from build123d import *

# Parameters (mm, degrees)
PAD_DEPTH       = 6
POCKET_DEPTH    = 5
SKETCH002_R     = 2.25
SKETCH002_R_2   = 1.6
PAD001_DEPTH    = 4
POCKET001_DEPTH = 10


with BuildPart() as part:
    # Sketch → Pad (new body)
    with BuildSketch(Plane.XY):
        with BuildLine():
            Line((3, 0), (62, 0))
            ThreePointArc((62, 0), (64.12132, 0.87868), (65, 3))
            Line((65, 3), (65, 27))
            ThreePointArc((65, 27), (64.12132, 29.12132), (62, 30))
            Line((62, 30), (3, 30))
            ThreePointArc((3, 30), (0.87868, 29.12132), (0, 27))
            Line((0, 27), (0, 3))
            ThreePointArc((0, 3), (0.87868, 0.87868), (3, 0))
        make_face()
    extrude(amount=PAD_DEPTH)

    # Sketch001 → Pocket (cut)
    with BuildSketch(Plane.XY):
        with BuildLine():
            Line((1, 27), (1, 3))
            ThreePointArc((1, 3), (1.585786, 1.585786), (3, 1))
            Line((3, 1), (62, 1))
            ThreePointArc((62, 1), (63.414214, 1.585786), (64, 3))
            Line((64, 3), (64, 27))
            ThreePointArc((64, 27), (63.414214, 28.414214), (62, 29))
            Line((62, 29), (3, 29))
            ThreePointArc((3, 29), (1.585786, 28.414214), (1, 27))
        make_face()
    extrude(amount=POCKET_DEPTH, mode=Mode.SUBTRACT)

    # Sketch002 → Pad001 (join)
    with BuildSketch(Plane.XY.offset(1)):
        with Locations((62.25, 27.3)):
            Circle(SKETCH002_R)
        with Locations((62.25, 27.3)):
            Circle(SKETCH002_R_2, mode=Mode.SUBTRACT)
        with Locations((2.75, 27.3)):
            Circle(SKETCH002_R)
        with Locations((2.75, 27.3)):
            Circle(SKETCH002_R_2, mode=Mode.SUBTRACT)
        with Locations((2.75, 2.7)):
            Circle(SKETCH002_R)
        with Locations((2.75, 2.7)):
            Circle(SKETCH002_R_2, mode=Mode.SUBTRACT)
        with Locations((62.25, 2.7)):
            Circle(SKETCH002_R)
        with Locations((62.25, 2.7)):
            Circle(SKETCH002_R_2, mode=Mode.SUBTRACT)
    extrude(amount=PAD001_DEPTH)

    # Sketch003 → Pocket001 (cut)
    with BuildSketch(Plane.YZ.offset(70)):
        with BuildLine():
            Line((10.57, 3.9), (10.57, 2.75))
            ThreePointArc((10.57, 2.75), (10.892183, 1.972183), (11.67, 1.65))
            Line((11.67, 1.65), (18.57, 1.65))
            ThreePointArc((18.57, 1.65), (19.347817, 1.972183), (19.67, 2.75))
            Line((19.67, 2.75), (19.67, 3.9))
            ThreePointArc((19.67, 3.9), (19.347817, 4.677817), (18.57, 5))
            Line((18.57, 5), (11.67, 5))
            ThreePointArc((11.67, 5), (10.892183, 4.677817), (10.57, 3.9))
        make_face()
    extrude(amount=-POCKET001_DEPTH, mode=Mode.SUBTRACT)


solid = part.part
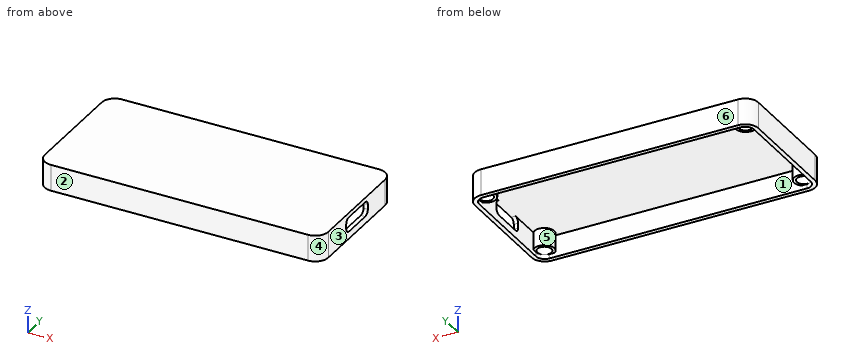
Read the model definition and answer for the solid it produces. Units are mm, in the model's axes. Face numbers are marked on the shaded views. A direction names the side the tool comes from. Round coordinates to 2 decimals unless told otherwise and drop trailing zeros. Write each loop counter-clockwise with the first axis right and the second up, starting at its lowest first coordinate (ties: lowest second). Pieces come first, ordered by that corner, then holes.
1. The part is cut by section B-B, the plane x = 37.5. Determine the outline of the cut face in (y, z).
2. Given pin 1 Ø2.5 at (x, y) = (3, 3) entering from -Z; pin 2 Ø3 at (x, y) = (2.75, 2.7) entering from -Z; pin 3 Ø1.1 at (x, z) = (64.5, 3) entering from +Y, each flat-ended and moving along its own axis, determine where each tip first touches the part or whether it passes through.
3. Determine the mould class of the marked faces 3, 4, 5 and 6 for opening direction Y: pulls with the +Y half, pulls with the -Y half, needs draft (parallel to the pull), parting line crosses it, or undercut.
4. The part is cut by section A-A, the plane y = 9.25. Determine the outline of the cut face in (x, z), then the cut area to 3 significant figures.
5. Straight lines are drawn through the part: L1, parallel to Y at x = 2.75, z = 3.05; L2, parallel to Y at x = 4.5, z = 3.2; L3, parallel to X at y = 5, z = 0.8. For each, find the intervals that lie inside material, in ascending order.
6. Which of the six approach directions +Z, -Z, +X, -X, +Y, -Y give full straight-line access (tool end or side, diameter ignored) to the marked faces 1 and 2?
Values:
1. outline: (0, 0) - (1, 0) - (1, 5) - (29, 5) - (29, 0) - (30, 0) - (30, 6) - (0, 6) - close
2. pin 1: stops at z = 1
2. pin 2: stops at z = 5
2. pin 3: stops at y = 29.28
3. face 3: needs draft
3. face 4: pulls with the -Y half
3. face 5: undercut
3. face 6: pulls with the +Y half
4. outline: (0, 0) - (1, 0) - (1, 5) - (64, 5) - (64, 0) - (65, 0) - (65, 6) - (0, 6) - close
4. area: 75.0 mm2
5. L1: y = 0.01 to 1.1, 4.3 to 4.95, 25.05 to 25.7, 28.9 to 29.99
5. L2: y = 0 to 1, 1.29 to 4.11, 25.89 to 28.71, 29 to 30
5. L3: x = 0 to 1, 64 to 65
6. face 1: -Z
6. face 2: +Z, -Z, +X, -X, -Y
